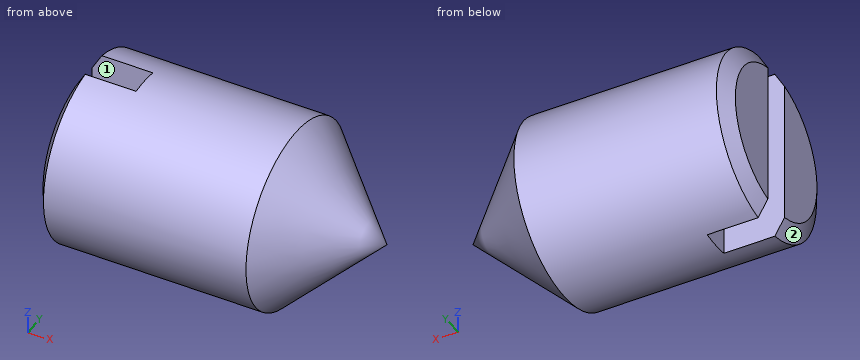
from build123d import *

# Parameters (mm, degrees)
SKETCH2_W  = 6
SKETCH2_H  = 1
SLOT_DEPTH = 2


with BuildPart() as part:
    # BodySke → BaseBody (revolve)
    with BuildSketch(Plane.XY):
        Polygon((0, 0), (0, 2.4455), (0.320140724, 3), (7, 3), (10, 0), align=None)
    revolve(axis=Axis((-12.7, 0, 0), (1, 0, 0)))

    # Sketch2 → Slot (cut)
    with BuildSketch(Plane.ZY):
        Rectangle(SKETCH2_W, SKETCH2_H)
    extrude(amount=-SLOT_DEPTH, mode=Mode.SUBTRACT)


solid = part.part
For this review, take the finished solid that the model builds, in its own axes (mm). Face numbers are marked on the shaded views. A direction names the side the tool comes from. Round coordinates to 2 decimals unless told otherwise and drop trailing zeros. Write each loop counter-clockwise with the first axis right and the second up, starting at its lowest first coordinate (ties: lowest second). Pieces come first, ordered by that corner, then holes. Notation, with made-up numbers: (82.25, -11) -> (112.25, -11) arc R13 ccw to (112.25, 13) -> close; hole circle Ø11 at (76, 88). An arc over 180 degrees is marked (long way). Use CSV: the item, a comma, the result in double quotes.
(1) Consider section A-A, the plane x = 4.5. Give the boundary of the cut face in (y, z).
Computed values:
outline,"circle Ø6 at (0, 0)"
(2) Clearance check with flat-ended pins moving along their axes: P1, Ø3, axis at x = 3, z = 2, coming from the -Y side; P2, Ø2, axis at x = 5, y = 1.5, coming from the -Z side; P3, Ø0.6, axis at x = 1, z = -1.5, coming from the -Y side. State where each tip first meets the part, or that it passes through.
Computed values:
P1,"y = -2.96"
P2,"z = -2.96"
P3,"y = -2.75"
(3) To check wall thickness, follow L1, parallel to Z at x = 6.75, y = 0.1; L2, parallel to Y at x = 1, z = -0.25; L3, parallel to Y at x = 2.5, z = 0.5. State the ranges of each line that lie inside material, in increasing order. Write a range as [from, to].
Computed values:
L1,"[-3, 3]"
L2,"[-2.99, -0.5], [0.5, 2.99]"
L3,"[-2.96, 2.96]"
(4) For the marked faces 1 and 2, list the 3-axis set-ups (+Z, -Z, +X, -X, +Y, -Y) from which the entire face can be reached by the end or side of a thin tool; tool diameter is ignored.
Computed values:
face 1,"+Z, -Z, -X"
face 2,"-X, -Y"
